Autodesk Inventor part; units mm, degrees
ref_plane "YZ Plane" through (0, 0, 0) normal (1, 0, 0) x (0, 1, 0)
ref_plane "XZ Plane" through (0, 0, 0) normal (0, 1, 0) x (-1, 0, 0)
ref_plane "XY Plane" through (0, 0, 0) normal (0, 0, 1) x (1, 0, 0)
sketch "Sketch1" plane through (0, 0, 0) normal (0, 0, 1) x (1, 0, 0)
  line L0 (-37.1271, 279.7291) -> (1.4084, 279.7291)
  line L1 (1.4084, 279.7291) -> (1.4084, -4.9324)
  line L2 (1.4084, -4.9324) -> (-37.1271, -4.9324)
  line L3 (-37.1271, -4.9324) -> (-37.1271, 279.7291)
  point P0 (0, 0)
  dimension "d0" = 38.5354
  dimension "d1" = 284.6614
extrude "Extrusion1" add sketch "Sketch1" along normal blind 108.8571
sketch "Sketch2" plane through (0, 0, 108.8571) normal (0, 0, 1) x (1, 0, 0)
  line L0 (-37.1271, -4.9324) -> (1.4084, -4.9324)
  line L1 (-17.8594, -4.9324) -> (-17.8594, 16.8391) construction
  circle A0 centre (-17.8594, 16.8391) radius 13.6071 construction
  line L2 (-17.8594, 16.8391) -> (-20.753, 30.135) construction
  line L3 (-17.8594, 16.8391) -> (-14.9657, 30.135) construction
  line L4 (-20.753, 30.135) -> (-14.9657, 30.135)
  line L5 (-17.8594, 16.8391) -> (-31.1553, 13.9454) construction
  line L6 (-31.1553, 13.9454) -> (-31.1553, 19.7327)
  line L7 (-17.8594, 16.8391) -> (-14.9657, 3.5432) construction
  line L8 (-14.9657, 3.5432) -> (-20.753, 3.5432)
  line L9 (-17.8594, 16.8391) -> (-4.5634, 19.7327) construction
  line L10 (-4.5634, 19.7327) -> (-4.5634, 13.9454)
  line L11 (-20.753, 30.135) -> (-20.753, 19.7327)
  line L12 (-20.753, 13.9454) -> (-20.753, 3.5432)
  line L13 (-31.1553, 13.9454) -> (-20.753, 13.9454)
  line L14 (-14.9657, 13.9454) -> (-4.5634, 13.9454)
  line L15 (-14.9657, 3.5432) -> (-14.9657, 13.9454)
  line L16 (-14.9657, 19.7327) -> (-14.9657, 30.135)
  line L17 (-14.9657, 19.7327) -> (-4.5634, 19.7327)
  line L18 (-31.1553, 19.7327) -> (-20.753, 19.7327)
  point P0 (0, 0)
  dimension "d4" = 21.7714
  dimension "d5" = 27.2143
  dimension "d18" = 360
fillet "Fillet1" radius 19.2677 2 edges at (1.4084, -4.9324, 54.4286) (-37.1271, -4.9324, 54.4286)
chamfer "Chamfer1" distance 19.2677 distance2 239.4857 1 edges at (-37.1271, 279.7291, 54.4286) measured on face at (-11.4368, 279.7291, 36.2857)
chamfer "Chamfer2" distance 239.4857 distance2 19.2677 1 edges at (1.4084, 279.7291, 54.4286) measured on face at (1.4084, 102.7999, 36.2857)
sketch "Sketch3" plane through (0, 0, 108.8571) normal (0, 0, 1) x (1, 0, 0)
  point P0 (0, 0)
extrude "Extrusion3" cut sketch "Sketch2" against normal blind 25.4
sketch "Sketch4" plane through (0, 0, 108.8571) normal (0, 0, 1) x (1, 0, 0)
  line L0 (-31.1553, 19.7327) -> (-31.1553, 13.9454)
  line L1 (-31.1553, 13.9454) -> (-31.1553, 19.7327)
  line L2 (-31.1553, 16.8391) -> (-13.0927, 16.8391) construction
  line L3 (-4.5634, 19.7327) -> (-14.9657, 19.7327)
  circle A0 centre (-17.8594, 16.8391) radius 4.0922
  point P0 (0, 0)
fillet "Fillet3" radius 0.6802 2 edges at (-17.8593, 279.7291, 54.4286) (-17.8594, 279.7291, 54.4286)
properties part number "Bistable Flipper 2" material "Stainless Steel, Polished"
Can you work these out from the model? Positions are in its coordinate system, mm. A direction names the side the tool comes from. Round coordinates to 2 decimals unless told otherwise and drop trailing zeros. Loops run counter-clockwise (first coordinate to the right, second up) from the corner with the lowest first, then second, coordinate; pieces in that order, holes last. Notation, with made-up numbers: (-21.5, -14.5) -> (37.5, -14.5) arc R9 ccw to (37.5, -3.5) -> close; hole circle Ø3 at (86.5, 24). An arc over 180 degrees is marked (long way). One line per item, written item: value. Start each with the question number.
1. If we mould it in two halves opening along X, with no side actions, what happens to faces 3 (the flat face through (-4.563, 17, 96)), 4 (the flat face through (-27.96, 154.16, 55.19)), 5 (the flat face through (1.408, 27, 54)), 6 (the flat face through (-26, 13.945, 96))? For each: pulls with the +X half, pulls with the -X half, needs draft (parallel to the pull), parting line crosses it, or undercut.
2. If we section it at D-D, the plane y = 152: Write out the boundary of the cut face in (x, z), then the cut area to 3 significant figures.
3. For pin 1 (3 mm diameter, centred on x = -7.5, z = 62, fed in from -Y); pin 2 (11.5 mm diameter, centred on y = 10, z = 90, fed in from -X); pin 3 (5 mm diameter, centred on x = -25.5, z = 100, fed in from -Y); pin 4 (11.5 mm diameter, centred on y = 7, z = 93.5, fed in from +X), each with a flat end and sliding along its axis, tell me the tip position at first contact or that it passes through.
4. If we section it at C-C, the plane x = -9: Write out the boundary of the cut face in (y, z), then the cut area to 3 significant figures.
5. If I drill on probe 1 along X at (y, z) = (258.5, 98); probe 2 along X at (y, z) = (233, 82.5), over which ranges is the centre line in solid material (lowest first)?
6. For faces 1 (the cylindrical face through (-31.63, 0.86, 55.19)), 2 (the flat face through (-18, 30.135, 96)), which set-ups out of +Z, -Z, +X, -X, +Y, -Y let a thin tool reach every point of the face, with its end or its side?
Calculated:
1. face 3: undercut
1. face 4: pulls with the -X half
1. face 5: pulls with the +X half
1. face 6: undercut
2. outline: (-28.14, 0) -> (-7.58, 0) -> (-7.58, 108.86) -> (-28.14, 108.86) -> close
2. area: 2,240 mm²
3. pin 1: stops at y = -2.77
3. pin 2: stops at x = -37.13
3. pin 3: stops at y = -4.23
3. pin 4: stops at x = 1.34
4. outline: (-2.77, 0) -> (169.61, 0) -> (169.61, 108.86) -> (19.73, 108.86) -> (19.73, 83.46) -> (13.95, 83.46) -> (13.95, 108.86) -> (-2.77, 108.86) -> close
4. area: 18,600 mm²
5. probe 1: x = -19.57 to -16.15
5. probe 2: x = -21.62 to -14.1
6. face 1: +Z, -Z, -X, -Y
6. face 2: +Z
